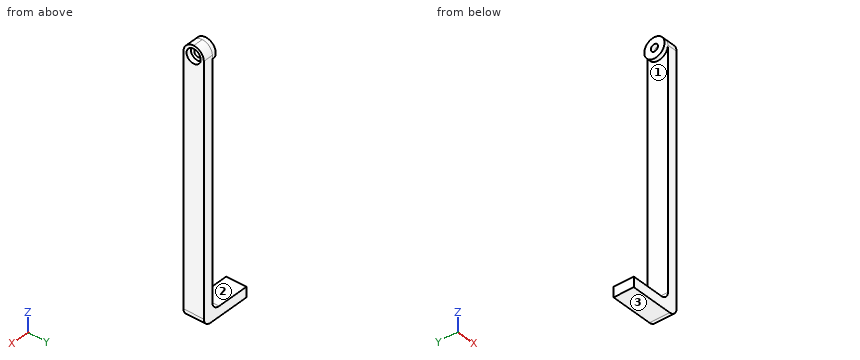
Autodesk Fusion 360 part; units mm, degrees
sketch "Sketch1" plane through (0, 0, 0) normal (0, 1, 0) x (1, 0, 0)
  line L0 (0, 0) -> (25, 0) construction
  line L1 (25, 0) -> (25, 130) construction
  line L2 (25, 130) -> (0, 130) construction
  line L3 (0, 130) -> (0, 0) construction
  line L4 (25, 0) -> (20, 0)
  line L5 (0, 130) -> (0, 125)
  line L6 (20, 121) -> (20, 0)
  line L7 (25, 0) -> (25, 126)
  line L8 (0, 130) -> (21, 130)
  line L9 (16, 125) -> (0, 125)
  arc A0 (20, 121) -> (16, 125) centre (16, 121) ccw
  arc A1 (25, 126) -> (21, 130) centre (21, 126) ccw
  dimension "d1" = 25
  dimension "d2" = 130
  dimension "d3" = 5
  dimension "d4" = 4
  dimension "d5" = 4
  dimension "d18" = 5
extrude "Extrude1" add sketch "Sketch1" along normal blind 10
fillet "Fillet1" radius 5 2 edges at (22.5, 10, 0) (22.5, 0, 0)
sketch "Sketch2" plane through (25, 0, 0) normal (1, 0, 0) x (0, 0, -1)
  arc A0 (5, 10) -> (5, 0) centre (5, 5) ccw
  line L0 (5, 0) -> (126, 0)
  line L1 (126, 0) -> (126, 10)
  line L2 (126, 10) -> (5, 10)
  line L3 (0, 5) -> (5, 5) construction
  circle A1 centre (5, 5) radius 1.75
  circle A2 centre (5, 5) radius 3.5
  dimension "d9" = 5
  dimension "d10" = 3.5
  dimension "d11" = 7
extrude "Extrude2" cut sketch "Sketch2" against normal up to surface (5 mm away) contours A1
extrude "Extrude3" cut sketch "Sketch2" against normal blind 2.5 contours A2
sketch "Sketch3" plane through (20, 0, 0) normal (-1, 0, 0) x (0, 0, 1)
  circle A0 centre (-5, 5) radius 1.75
  arc A1 (-5, 0) -> (-5, 10) centre (-5, 5) ccw
  line L0 (-5, 10) -> (-121, 10)
  line L1 (-121, 10) -> (-121, 0)
  line L2 (-121, 0) -> (-5, 0)
  circle A2 centre (-5, 5) radius 5
extrude "Extrude4" add sketch "Sketch3" along normal blind 2 contours A1 A2
Could you check a few things on this model? Use its own coordinates, in mm. Face numbers are marked on the shaded views. Round coordinates to 2 decimals unless told otherwise and drop trailing zeros. Loops run counter-clockwise (first coordinate to the right, second up) from the corner with the lowest first, then second, coordinate; pieces in that order, holes last. Notation, with made-up numbers: M -8,15 L 10,15 A13 ccw 10,22 Z; hole C 85,27.5 d1. An arc over 180 degrees is marked long. Put each result on its own line as item: value.
Q1. I need wall thicknesses on probe 1 along Y at (x, z) = (20.95, -5); probe 2 along X at (y, z) = (7.25, -56); probe 3 along Z at (x, y) = (10, 3). Which ranges of each line are inside material? Lowest first, please.
Check result:
probe 1: 0 to 3.25, 6.75 to 10
probe 2: 20 to 25
probe 3: -130 to -125
Q2. Imagine slicing it at B-B (x = 3). Write out the boundary of the cut face in (y, z), then the cut area to 3 significant figures.
Check result:
outline: M 0,-130 L 10,-130 L 10,-125 L 0,-125 Z
area: 50.0 mm2
Q3. Thinking about a two-plate mould opening in Z: for the marked faces 1, 2 and 3, which applies, released by +Z, released by -Z, zero draft, split by the parting line, or undercut?
Check result:
face 1: undercut
face 2: released by +Z
face 3: released by -Z
Q4. Imagine slicing it at A-A (z = -114.5). Write out the boundary of the cut face in (x, y).
Check result:
outline: M 20,0 L 25,0 L 25,10 L 20,10 Z
Q5. For pin 1 (5 mm diameter, centred on y = 3.5, z = -5, fed in from -X); pin 2 (2 mm diameter, centred on x = 14.5, y = 2, fed in from +Z); pin 3 (6 mm diameter, centred on y = 8.5, z = -15, fed in from -X), each with a flat end and sliding along its axis, tell me the tip position at first contact or that it passes through.
Check result:
pin 1: x = 18
pin 2: z = -125
pin 3: x = 20
